Can you work these out from the model? Positions are in its coordinate system, mm. Face numbers are marked on the shaded views. A direction names the side the tool comes from. Coordinates: 2 decimals unless noted, no trailing zeros. Loops run counter-clockwise (first coordinate to the right, second up) from the corner with the lowest first, then second, coordinate; pieces in that order, holes last.
```python
from build123d import *

# Parameters (mm, degrees)
ESQUISSE1_W             = 45
ESQUISSE1_H             = 30
BOSS_EXTRU_1_DEPTH      = 8
ESQUISSE5_W             = 30
ESQUISSE5_H             = 48
BOSS_EXTRU_3_DEPTH      = 45
ENL_V_MAT_EXTRU_1_DEPTH = 27
CONG_1_R                = 2
ESQUISSE16_R            = 3.5
BOSS_EXTRU_5_DEPTH      = 9
D_GAGEMENT_M32_D        = 3.2
D_GAGEMENT_M33_D        = 3.2
D_GAGEMENT_M33_DEPTH    = 8
D_GAGEMENT_M33_TIP      = 0.96137699
ESQUISSE28_W            = 10
ESQUISSE28_H            = 12
ENL_V_MAT_EXTRU_2_DEPTH = 70.045275001


with BuildPart() as part:
    # Esquisse1 → Boss.-Extru.1 (new body)
    with BuildSketch(Plane(origin=(0, 0, 0), x_dir=(1, 0, 0), z_dir=(0, 1, 0))):
        with Locations((6, 0)):
            Rectangle(ESQUISSE1_W, ESQUISSE1_H)
    extrude(amount=BOSS_EXTRU_1_DEPTH)

    # Esquisse5 → Boss.-Extru.3 (add)
    with BuildSketch(Plane.ZY.offset(16.5)):
        with Locations((0, 32)):
            Rectangle(ESQUISSE5_W, ESQUISSE5_H)
    extrude(amount=-BOSS_EXTRU_3_DEPTH)

    # Esquisse6 → Enlèv. mat.-Extru.1 (cut)
    with BuildSketch(Plane.ZY.offset(16.5)):
        Polygon((10.5, 48), (4.5, 48), (4.5, 56), (-4.5, 56), (-4.5, 48), (-10.5, 48), (-10.5, 8), (10.5, 8), align=None)
    extrude(amount=-ENL_V_MAT_EXTRU_1_DEPTH, mode=Mode.SUBTRACT)

    # Congé1
    cong_1_edges = [part.edges().sort_by_distance(p)[0] for p in [
        (6, 56, -15),
        (6, 56, 15),
        (-16.5, 56, 9.75),
        (28.5, 56, 0),
        (-16.5, 56, -9.75),
        (10.5, 56, 0),
        (-3, 56, -4.5),
        (-3, 56, 4.5),
        (28.5, 28, 15),
        (-16.5, 28, 15),
        (-16.5, 28, -15),
        (28.5, 28, -15),
    ]]
    fillet(cong_1_edges, radius=CONG_1_R)

    # Esquisse16 → Boss.-Extru.5 (add)
    with BuildSketch(Plane(origin=(28.5, 0, 0), x_dir=(0, 0, -1), z_dir=(1, 0, 0))):
        with Locations(Location((0, 38, 0), (0, 0, 180))):
            Circle(ESQUISSE16_R)
    extrude(amount=BOSS_EXTRU_5_DEPTH)

    # Dégagement M32 (through all)
    with Locations(Plane(origin=(0, 8, 0), x_dir=(1, 0, 0), z_dir=(0, 1, 0))):
        with Locations((-7.5, 0), (7.5, 0)):
            Hole(D_GAGEMENT_M32_D / 2)

    # Dégagement M33
    with Locations(Plane.ZY.offset(16.5)):
        with Locations((-5, 3.5), (5, 3.5)):
            Hole(D_GAGEMENT_M33_D / 2, depth=D_GAGEMENT_M33_DEPTH)
            with Locations((0, 0, -(D_GAGEMENT_M33_DEPTH + D_GAGEMENT_M33_TIP / 2))):  # 118° drill point
                Cone(0, D_GAGEMENT_M33_D / 2, D_GAGEMENT_M33_TIP, mode=Mode.SUBTRACT)

    # Esquisse28 → Enlèv. mat.-Extru.2 (cut, through all)
    with BuildSketch(Plane(origin=(0, 56, 0), x_dir=(1, 0, 0), z_dir=(0, 1, 0))):
        with Locations((18.5, 0)):
            Rectangle(ESQUISSE28_W, ESQUISSE28_H)
    extrude(amount=-ENL_V_MAT_EXTRU_2_DEPTH, mode=Mode.SUBTRACT)


solid = part.part
```
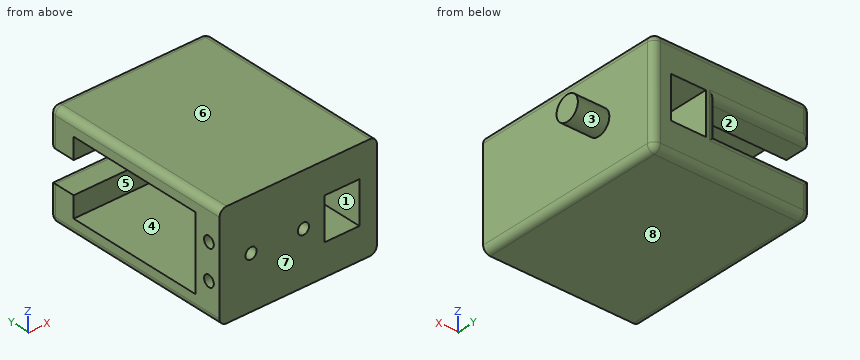
Item 1: On a 3-axis mill with a long thin cutter (end or side, diameter ignored), from which of +Z, -Z, +X, -X, +Y, -Y can I reach the whole of each face in a straight line? I mean the marked faces 1, 2, 3 and 4. Say none if no direction works.
Results are:
face 1: +Y, -Y
face 2: -X, +Y
face 3: +X
face 4: -X
Item 2: I'm going to push flat-ended pins straight in: P1, Ø3, axis at x = -7.5, z = 0, coming from the +Y side; P2, Ø2.5, axis at y = 3.5, z = 5, coming from the -X side; P3, Ø6, axis at y = 11.5, z = 7.5, coming from the +X side; P4, Ø1, axis at y = 31.5, z = -6.5, coming from the -X side. Where does each tip first touch, or does it pass through?
Results are:
P1: passes through
P2: stops at x = -8.29
P3: stops at x = 28.5
P4: stops at x = 10.5
Item 3: I need wall thicknesses on line 1 along Z through (x, y) = (-14.25, 3.5); line 2 along Y through (x, z) = (6, -10); line 3 along X through (y, z) = (15, -2.75). Which ranges of each line are inside material? Lowest first, please.
Results are:
line 1: z = -15 to -6.6, -3.4 to 3.4, 6.6 to 15
line 2: y = 0 to 8, 48 to 56
line 3: x = 10.5 to 13.5, 23.5 to 28.5
Item 4: Suppose I cut it at C-C, the plane y = 38. Please give me the cut outline in (x, z), plus the area to 3 significant figures.
Results are:
outline: (-16.5, -13) arc R2 ccw to (-14.5, -15) - (26.5, -15) arc R2 ccw to (28.5, -13) - (28.5, -3.5) - (37.5, -3.5) - (37.5, 3.5) - (28.5, 3.5) - (28.5, 13) arc R2 ccw to (26.5, 15) - (-14.5, 15) arc R2 ccw to (-16.5, 13) - (-16.5, 10.5) - (10.5, 10.5) - (10.5, -10.5) - (-16.5, -10.5) - close; hole (13.5, -6) - (23.5, -6) - (23.5, 6) - (13.5, 6) - close
area: 723 mm2
Item 5: Suppose I cut it at A-A, the plane x = 7.5. Please give me the cut outline in (y, z), plus the area to 3 significant figures.
Results are:
outline: (0, -15) - (54, -15) arc R2 ccw to (56, -13) - (56, -6.5) arc R2 ccw to (54, -4.5) - (48, -4.5) - (48, -10.5) - (8, -10.5) - (8, -1.6) - (0, -1.6) - close; (0, 1.6) - (8, 1.6) - (8, 10.5) - (48, 10.5) - (48, 4.5) - (54, 4.5) arc R2 ccw to (56, 6.5) - (56, 13) arc R2 ccw to (54, 15) - (0, 15) - close
area: 739 mm2
Item 6: We'd pull the mould along Z, two halves only. Please class the marked faces 5, 6, 7 and 8: +Z half, -Z half, draft (parallel to the pull), parting line (faces both ways), or undercut.
Results are:
face 5: undercut
face 6: +Z half
face 7: draft
face 8: -Z half
Item 7: Suppose I cut it at B-B, the plane z = 0. Please give me the cut outline in (x, y), plus the area to 3 significant figures.
Results are:
outline: (-16.5, 0) - (-9.1, 0) - (-9.1, 8) - (-16.5, 8) - close; (-5.9, 0) - (5.9, 0) - (5.9, 8) - (-5.9, 8) - close; (9.1, 0) - (13.5, 0) - (13.5, 56) - (12.5, 56) arc R2 ccw to (10.5, 54) - (10.5, 8) - (9.1, 8) - close; (23.5, 0) - (28.5, 0) - (28.5, 34.5) - (37.5, 34.5) - (37.5, 41.5) - (28.5, 41.5) - (28.5, 54) arc R2 ccw to (26.5, 56) - (23.5, 56) - close
area: 674 mm2
Item 8: Suppose I cut it at D-D, the plane x = -13. Please give me the cut outline in (y, z), plus the area to 3 significant figures.
Results are:
outline: (0, -15) - (54, -15) arc R2 ccw to (56, -13) - (56, -6.5) arc R2 ccw to (54, -4.5) - (48, -4.5) - (48, -10.5) - (8, -10.5) - (8, 10.5) - (48, 10.5) - (48, 4.5) - (54, 4.5) arc R2 ccw to (56, 6.5) - (56, 13) arc R2 ccw to (54, 15) - (0, 15) - close; hole circle Ø3.2 at (3.5, -5); hole circle Ø3.2 at (3.5, 5)
area: 748 mm2
